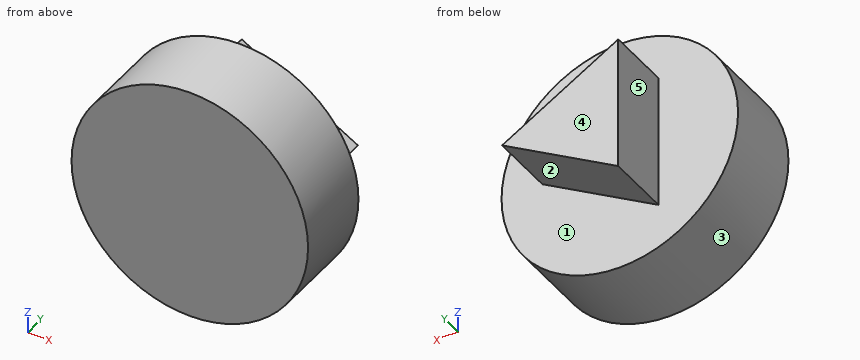
from build123d import *

# Parameters (mm, degrees)
SKETCH1_R           = 7.25
BOSS_EXTRUDE1_DEPTH = 5
BOSS_EXTRUDE2_DEPTH = 4


with BuildPart() as part:
    # Sketch1 → Boss-Extrude1 (new body)
    with BuildSketch(Plane(origin=(0, 0, 0), x_dir=(1, 0, 0), z_dir=(0, 1, 0))):
        with Locations(Location((0, 0, 0), (0, 0, 270))):
            Circle(SKETCH1_R)
    extrude(amount=BOSS_EXTRUDE1_DEPTH)

    # Sketch2 → Boss-Extrude2 (add)
    with BuildSketch(Plane(origin=(0, 5, 0), x_dir=(1, 0, 0), z_dir=(0, 1, 0))):
        Polygon((4.75, 0), (-2.375, 4.113620668), (-2.375, -4.113620668), align=None)
    extrude(amount=BOSS_EXTRUDE2_DEPTH)


solid = part.part
The model under review builds one solid part; all positions refer to its coordinate system, in mm. Face numbers are marked on the shaded views. A direction names the side the tool comes from. Give positions to 0.01 mm unless a question says otherwise; leave off trailing zeros. Order: outer loops, then holes, each group sorted by start corner. A loop starts at its lowest first (then second) coordinate and runs counter-clockwise, first axis right, second up. Notation, with made-up numbers: (-29.5, 72.25) -> (2.5, 72.25) arc R27 cw to (2.5, 92.25) -> close; hole circle Ø11 at (-19, -33). An arc over 180 degrees is marked (long way). Write item = value, one per line. Start each with the question number.
(1) For L1, parallel to Y at x = -4, z = 5; L2, parallel to X at y = 2, z = -0.25; L3, parallel to Z at x = 1.25, y = 3.25, list the stretches that pass through material, from the lowest coordinate up. Write a range as from..to.
(2) For pin 1 Ø2 at (y, z) = (2.5, 1.5) entering from +X; pin 2 Ø1.2 at (y, z) = (8, -2) entering from -X (3 decimals); pin 3 Ø2 at (y, z) = (4, -3.5) entering from -X, all flat-tipped, find the tip position at first contact; note any pin that passes through.
(3) Take a section at A-A (x = -1). Write out the cut boundary in (y, z), plus the area to 3 significant figures.
(4) Draft analysis for pull direction X (two halves, no side actions). For the marked faces 1, 2 and 3, state which applies: +X half, -X half, draft (parallel to the pull), parting line (faces both ways), or undercut.
(5) Tool access review of the marked faces 4 and 5: name each direction out of +Z, -Z, +X, -X, +Y, -Y from which nothing blocks a thin tool from reaching the whole face with its end or side.
(6) Take a section at D-D (x = -5). Write out the cut boundary in (y, z), plus the area to 3 significant figures.
(7) Take a section at B-B (z = -0.75). Write out the cut boundary in (x, y) (3 decimals), plus the area to 3 significant figures.
(8) Take a section at C-C (y = 2). Write out the cut boundary in (x, z).
Returned:
q1.L1 = 0..5
q1.L2 = -7.25..7.25
q1.L3 = -7.14..7.14
q2.pin_1 = 7.23
q2.pin_2 = -2.375
q2.pin_3 = -6.81
q3.outline = (0, -7.18) -> (5, -7.18) -> (5, -3.32) -> (9, -3.32) -> (9, 3.32) -> (5, 3.32) -> (5, 7.18) -> (0, 7.18) -> close
q3.area = 98.4 mm²
q4.face_1 = draft
q4.face_2 = +X half
q4.face_3 = parting line
q5.face_4 = +Z, -Z, +X, -X, +Y
q5.face_5 = +Z, -Z, -X, +Y
q6.outline = (0, -5.25) -> (5, -5.25) -> (5, 5.25) -> (0, 5.25) -> close
q6.area = 52.5 mm²
q7.outline = (-7.211, 0) -> (7.211, 0) -> (7.211, 5) -> (3.451, 5) -> (3.451, 9) -> (-2.375, 9) -> (-2.375, 5) -> (-7.211, 5) -> close
q7.area = 95.4 mm²
q8.outline = circle Ø14.5 at (0, 0)
